Geometry check sheet. Reference: the model listing, model coordinates, mm. Face numbers are marked on the shaded views. Round coordinates to 2 decimals unless told otherwise and drop trailing zeros. Order: outer loops, then holes, each group sorted by start corner. A loop starts at its lowest first (then second) coordinate and runs counter-clockwise, first axis right, second up.
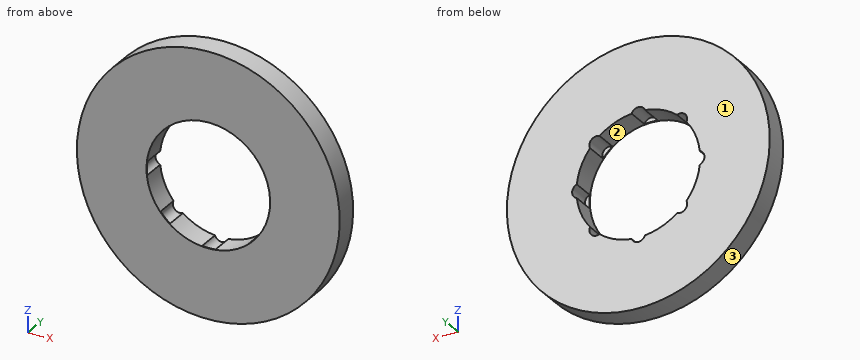
```python
from build123d import *

# Parameters (mm, degrees)
SKETCH1_R           = 85
BOSS_EXTRUDE1_DEPTH = 15
SKETCH2_R           = 40
CUT_EXTRUDE1_DEPTH  = 122.140414396
SKETCH3_R           = 4.608597006
CUT_EXTRUDE2_DEPTH  = 14.406553
CIRPATTERN1_START   = 0.593447211
CIRPATTERN1_DEPTH   = 14.406552789


# Read off the part's stored shape, not the designer's step: CirPattern1
with BuildPart() as part:
    # Sketch1 → Boss-Extrude1 (new body)
    with BuildSketch(Plane(origin=(0, 0, 0), x_dir=(1, 0, 0), z_dir=(0, 1, 0))):
        with Locations(Location((0, 0, 0), (0, 0, 270))):
            Circle(SKETCH1_R)
    extrude(amount=BOSS_EXTRUDE1_DEPTH)

    # Sketch2 → Cut-Extrude1 (cut, through all)
    with BuildSketch(Plane(origin=(0, 0, 0), x_dir=(1, 0, 0), z_dir=(0, 1, 0))):
        with Locations(Location((0, 0, 0), (0, 0, 270))):
            Circle(SKETCH2_R)
    extrude(amount=CUT_EXTRUDE1_DEPTH, mode=Mode.SUBTRACT)

    # Sketch3 → Cut-Extrude2 (cut)
    with BuildSketch(Plane(origin=(0, 15, 0), x_dir=(1, 0, 0), z_dir=(0, 1, 0))):
        with Locations((-38.186141272, 0)):
            Circle(SKETCH3_R)
    extrude(amount=-CUT_EXTRUDE2_DEPTH, mode=Mode.SUBTRACT)

    # CirPattern1 outline → CirPattern1 (cut)
    with BuildSketch(Plane(origin=(0, 0, 0), x_dir=(1, 0, 0), z_dir=(0, 1, 0)).offset(CIRPATTERN1_START)):
        with BuildLine():
            ThreePointArc((-25.056515086, -31.179657659), (-28.284271247, -28.284271247), (-31.179657659, -25.056515086))
            ThreePointArc((-31.179657659, -25.056515086), (-30.260449635, -30.260449635), (-25.056515086, -31.179657659))
        make_face()
        with BuildLine():
            ThreePointArc((-25.056515086, 31.179657659), (-30.260449635, 30.260449635), (-31.179657659, 25.056515086))
            ThreePointArc((-31.179657659, 25.056515086), (-28.284271247, 28.284271247), (-25.056515086, 31.179657659))
        make_face()
        with BuildLine():
            ThreePointArc((4.329715636, -39.764979096), (0, -40), (-4.329715636, -39.764979096))
            ThreePointArc((-4.329715636, -39.764979096), (0, -42.794738278), (4.329715636, -39.764979096))
        make_face()
        with BuildLine():
            ThreePointArc((4.329715636, 39.764979096), (0, 42.794738278), (-4.329715636, 39.764979096))
            ThreePointArc((-4.329715636, 39.764979096), (0, 40), (4.329715636, 39.764979096))
        make_face()
        with BuildLine():
            ThreePointArc((31.179657659, -25.056515086), (28.284271247, -28.284271247), (25.056515086, -31.179657659))
            ThreePointArc((25.056515086, -31.179657659), (30.260449635, -30.260449635), (31.179657659, -25.056515086))
        make_face()
        with BuildLine():
            ThreePointArc((31.179657659, 25.056515086), (30.260449635, 30.260449635), (25.056515086, 31.179657659))
            ThreePointArc((25.056515086, 31.179657659), (28.284271247, 28.284271247), (31.179657659, 25.056515086))
        make_face()
        with BuildLine():
            ThreePointArc((39.764979096, 4.329715636), (40, 0), (39.764979096, -4.329715636))
            ThreePointArc((39.764979096, -4.329715636), (42.794738278, 0), (39.764979096, 4.329715636))
        make_face()
    extrude(amount=CIRPATTERN1_DEPTH, mode=Mode.SUBTRACT)


solid = part.part
```
(1) Draft check along Z on the marked faces 1, 2 and 3. Enter one of: released by +Z, released by -Z, zero draft, split by the parting line, or undercut.
Returned:
face 1: zero draft
face 2: undercut
face 3: split by the parting line
(2) Depth check by flat-ended pin: P1, Ø4, axis at y = 6.5, z = 8.5, coming from the +X side; P2, Ø3.5, axis at x = 29, z = -27, coming from the +Y side; P3, Ø2, axis at y = 10.5, z = 64.5, coming from the -X side. Enter the tip coordinate at first touch or a pass-through.
Returned:
P1: stops at x = 84.75
P2: stops at y = 0.59
P3: stops at x = -56.5
(3) Sectioned sample at D-D, the plane x = 21. Record the cut outline in (y, z), and give its area (3 significant figures).
Returned:
outline: (0, -82.37) - (15, -82.37) - (15, -34.04) - (0, -34.04) - close; (0, 34.04) - (15, 34.04) - (15, 82.37) - (0, 82.37) - close
area: 1,450 mm2
(4) Sectioned sample at B-B, the plane z = 0. Record the cut outline in (x, y), and give its area (3 significant figures).
Returned:
outline: (-85, 0) - (-40, 0) - (-40, 0.59) - (-42.79, 0.59) - (-42.79, 15) - (-85, 15) - close; (40, 0) - (85, 0) - (85, 15) - (42.79, 15) - (42.79, 0.59) - (40, 0.59) - close
area: 1,270 mm2
(5) Sectioned sample at C-C, the plane y = 8.25. Record the cut outline in (x, z), and give its area (3 significant figures).
Returned:
outline: circle Ø170 at (0, 0); hole (-39.76, -4.33) arc R40 ccw to (-31.18, -25.06) arc R4.61 ccw to (-25.06, -31.18) arc R40 ccw to (-4.33, -39.76) arc R4.61 ccw to (4.33, -39.76) arc R40 ccw to (25.06, -31.18) arc R4.61 ccw to (31.18, -25.06) arc R40 ccw to (39.76, -4.33) arc R4.61 ccw to (39.76, 4.33) arc R40 ccw to (31.18, 25.06) arc R4.61 ccw to (25.06, 31.18) arc R40 ccw to (4.33, 39.76) arc R4.61 ccw to (-4.33, 39.76) arc R40 ccw to (-25.06, 31.18) arc R4.61 ccw to (-31.18, 25.06) arc R40 ccw to (-39.76, 4.33) arc R4.61 ccw to start
area: 17,500 mm2
(6) Sectioned sample at A-A, the plane x = 0. Record the cut outline in (y, z).
Returned:
outline: (0, -85) - (15, -85) - (15, -42.79) - (0.59, -42.79) - (0.59, -40) - (0, -40) - close; (0, 40) - (0.59, 40) - (0.59, 42.79) - (15, 42.79) - (15, 85) - (0, 85) - close
(7) Material ranges on line 1 (X direction, y = 5.5, z = 0); line 2 (X direction, y = 1, z = 15); line 3 (Z direction, x = 10, y = 4), recorded low to high.
Returned:
line 1: x = -85 to -42.79, 42.79 to 85
line 2: x = -83.67 to -37.08, 37.08 to 83.67
line 3: z = -84.41 to -38.73, 38.73 to 84.41
